```python
from build123d import *

# Parameters (mm, degrees)
F0_W     = 84
F0_H     = 93.5
F1_DEPTH = 4
F2_W     = 4
F2_H     = 4
F2_H_2   = 5.5
F3_DEPTH = 4
F5_DEPTH = 4
F6_W     = 13
F6_H     = 8
F7_DEPTH = 4
F9_DEPTH = 4


with BuildPart() as f1:
    # F0 (on Top) → F1 (new body)
    with BuildSketch(Plane.XY):
        with Locations((42, 46.75)):
            Rectangle(F0_W, F0_H)
    extrude(amount=F1_DEPTH)

    # F2 (on face) → F3 (cut, through all)
    with BuildSketch(Plane.XY.offset(4)):
        with Locations((2, 2)):
            Rectangle(F2_W, F2_H)
        with Locations((82, 2)):
            Rectangle(F2_W, F2_H)
        with Locations((2, 90.75)):
            Rectangle(F2_W, F2_H_2)
        with Locations((82, 90.75)):
            Rectangle(F2_W, F2_H_2)
    extrude(amount=-F3_DEPTH, mode=Mode.SUBTRACT)

    # F4 (on face) → F5 (cut, through all)
    with BuildSketch(Plane.XY.offset(4)):
        with BuildLine():
            ThreePointArc((10.5, 83.5), (9.792893, 83.207107), (9.5, 82.5))
            Line((9.5, 82.5), (9.5, 11))
            ThreePointArc((9.5, 11), (9.792893, 10.292893), (10.5, 10))
            ThreePointArc((10.5, 10), (11.207107, 10.292893), (11.5, 11))
            Line((11.5, 11), (11.5, 82.5))
            ThreePointArc((11.5, 82.5), (11.207107, 83.207107), (10.5, 83.5))
        make_face()
        with BuildLine():
            ThreePointArc((17.5, 83.5), (16.792893, 83.207107), (16.5, 82.5))
            Line((16.5, 82.5), (16.5, 11))
            ThreePointArc((16.5, 11), (16.792893, 10.292893), (17.5, 10))
            ThreePointArc((17.5, 10), (18.207107, 10.292893), (18.5, 11))
            Line((18.5, 11), (18.5, 82.5))
            ThreePointArc((18.5, 82.5), (18.207107, 83.207107), (17.5, 83.5))
        make_face()
        with BuildLine():
            ThreePointArc((24.5, 83.5), (23.792893, 83.207107), (23.5, 82.5))
            Line((23.5, 82.5), (23.5, 11))
            ThreePointArc((23.5, 11), (23.792893, 10.292893), (24.5, 10))
            ThreePointArc((24.5, 10), (25.207107, 10.292893), (25.5, 11))
            Line((25.5, 11), (25.5, 82.5))
            ThreePointArc((25.5, 82.5), (25.207107, 83.207107), (24.5, 83.5))
        make_face()
        with BuildLine():
            ThreePointArc((31.5, 83.5), (30.792893, 83.207107), (30.5, 82.5))
            Line((30.5, 82.5), (30.5, 11))
            ThreePointArc((30.5, 11), (30.792893, 10.292893), (31.5, 10))
            ThreePointArc((31.5, 10), (32.207107, 10.292893), (32.5, 11))
            Line((32.5, 11), (32.5, 82.5))
            ThreePointArc((32.5, 82.5), (32.207107, 83.207107), (31.5, 83.5))
        make_face()
        with BuildLine():
            ThreePointArc((38.5, 83.5), (37.792893, 83.207107), (37.5, 82.5))
            Line((37.5, 82.5), (37.5, 11))
            ThreePointArc((37.5, 11), (37.792893, 10.292893), (38.5, 10))
            ThreePointArc((38.5, 10), (39.207107, 10.292893), (39.5, 11))
            Line((39.5, 11), (39.5, 82.5))
            ThreePointArc((39.5, 82.5), (39.207107, 83.207107), (38.5, 83.5))
        make_face()
        with BuildLine():
            ThreePointArc((45.5, 83.5), (44.792893, 83.207107), (44.5, 82.5))
            Line((44.5, 82.5), (44.5, 11))
            ThreePointArc((44.5, 11), (44.792893, 10.292893), (45.5, 10))
            ThreePointArc((45.5, 10), (46.207107, 10.292893), (46.5, 11))
            Line((46.5, 11), (46.5, 82.5))
            ThreePointArc((46.5, 82.5), (46.207107, 83.207107), (45.5, 83.5))
        make_face()
        with BuildLine():
            ThreePointArc((52.5, 83.5), (51.792893, 83.207107), (51.5, 82.5))
            Line((51.5, 82.5), (51.5, 11))
            ThreePointArc((51.5, 11), (51.792893, 10.292893), (52.5, 10))
            ThreePointArc((52.5, 10), (53.207107, 10.292893), (53.5, 11))
            Line((53.5, 11), (53.5, 82.5))
            ThreePointArc((53.5, 82.5), (53.207107, 83.207107), (52.5, 83.5))
        make_face()
        with BuildLine():
            ThreePointArc((59.5, 83.5), (58.792893, 83.207107), (58.5, 82.5))
            Line((58.5, 82.5), (58.5, 11))
            ThreePointArc((58.5, 11), (58.792893, 10.292893), (59.5, 10))
            ThreePointArc((59.5, 10), (60.207107, 10.292893), (60.5, 11))
            Line((60.5, 11), (60.5, 82.5))
            ThreePointArc((60.5, 82.5), (60.207107, 83.207107), (59.5, 83.5))
        make_face()
        with BuildLine():
            ThreePointArc((66.5, 83.5), (65.792893, 83.207107), (65.5, 82.5))
            Line((65.5, 82.5), (65.5, 11))
            ThreePointArc((65.5, 11), (65.792893, 10.292893), (66.5, 10))
            ThreePointArc((66.5, 10), (67.207107, 10.292893), (67.5, 11))
            Line((67.5, 11), (67.5, 82.5))
            ThreePointArc((67.5, 82.5), (67.207107, 83.207107), (66.5, 83.5))
        make_face()
        with BuildLine():
            ThreePointArc((73.5, 83.5), (72.792893, 83.207107), (72.5, 82.5))
            Line((72.5, 82.5), (72.5, 11))
            ThreePointArc((72.5, 11), (72.792893, 10.292893), (73.5, 10))
            ThreePointArc((73.5, 10), (74.207107, 10.292893), (74.5, 11))
            Line((74.5, 11), (74.5, 82.5))
            ThreePointArc((74.5, 82.5), (74.207107, 83.207107), (73.5, 83.5))
        make_face()
    extrude(amount=-F5_DEPTH, mode=Mode.SUBTRACT)

    # F6 (on face) → F7 (join)
    with BuildSketch(Plane.XY.offset(4)):
        with Locations((90.5, 8)):
            Rectangle(F6_W, F6_H)
        with Locations((-6.5, 8)):
            Rectangle(F6_W, F6_H)
    extrude(amount=-F7_DEPTH)

    # F8 (on face) → F9 (join)
    with BuildSketch(Plane.XY.offset(4)):
        Polygon((93, 16), (93, 12), (97, 12), (95, 16), align=None)
        Polygon((93, 4), (93, 0), (95, 0), (97, 4), align=None)
        Polygon((-11, 16), (-13, 12), (-9, 12), (-9, 16), align=None)
        Polygon((-11, 0), (-9, 0), (-9, 4), (-13, 4), align=None)
    extrude(amount=-F9_DEPTH)


solid = f1.part
```
Source: CAD feature listing. Evaluate the final solid. Frame: model axes, mm. A direction names the side the tool comes from. Coordinates: 2 decimals unless noted, no trailing zeros. Loops run counter-clockwise (first coordinate to the right, second up) from the corner with the lowest first, then second, coordinate; pieces in that order, holes last. Notation, with made-up numbers: M 23,22 L 37,22 A22 cw 37,40 Z; hole C 82,44 d2. An arc over 180 degrees is marked long. Put each result on its own line as item: value. Start each with the question number.
1) Reachability of faces 1 (the face through (-9, 2, 2)), 2 (the face through (88, 12, 2)), 3 (the face through (30.5, 47, 2)) from +Z, -Z, +X, -X, +Y, -Y: full face, straight path, thin tool, end or side. Return the list, or none.
2) Ray query, L1, parallel to Y at x = 91.5, z = 0.5; L2, parallel to X at y = 84, z = 0.5. Return the intervals inside material, ascending. Write a range as from..to.
3) Pull-direction query (X, two-part tool) for faces 4 (the face through (74.5, 46, 2)), 5 (the face through (96, 14, 2)), 6 (the face through (-12, 14, 2)); classes: pulls with the +X half, pulls with the -X half, needs draft (parallel to the pull), parting line crosses it, or undercut.
4) Cut plane A-A on y = 64.5. Give the number of separate pieces and of enclosed holes in the cut face, then the cut area to 3 significant figures.
5) Cut plane D-D on x = 85.5. Return the cut outline in (y, z), then the cut area to 3 significant figures.
6) Contact query for flat-ended pins moving along their axis: pin 1 Ø1.6 at (x, z) = (-10, 1.5) entering from +Y; pin 2 Ø1.2 at (x, z) = (-2.5, 2) entering from +Y; pin 3 Ø2 at (y, z) = (2.5, 2.5) entering from +X. Output: stop coordinate, or through.
The answers:
1. face 1: +Z, -Z, -Y
1. face 2: +Z, -Z, +Y
1. face 3: +Z, -Z
2. L1: y = 4..12
2. L2: x = 0..84
3. face 4: undercut
3. face 5: pulls with the +X half
3. face 6: pulls with the -X half
4. separate pieces: 11
4. enclosed holes: 0
4. area: 256 mm²
5. outline: M 4,0 L 12,0 L 12,4 L 4,4 Z
5. area: 32.0 mm²
6. pin 1: stops at y = 16
6. pin 2: stops at y = 12
6. pin 3: stops at x = 96.75
